Autodesk Inventor part; units mm, degrees
ref_plane "Work Plane1" through (18.5, 0, 8) normal (0, 0, 1) x (1, 0, 0)
ref_plane "YZ Plane" through (0, 0, 0) normal (1, 0, 0) x (0, 1, 0)
ref_plane "XZ Plane" through (0, 0, 0) normal (0, 1, 0) x (-1, 0, 0)
sketch "Sketch1" plane through (0, 0, 0) normal (0, 0, 1) x (1, 0, 0)
  line L0 (0, 0) -> (88, 0)
  line L1 (88, 0) -> (88, 23)
  line L2 (88, 23) -> (72, 23)
  line L3 (72, 23) -> (72, 10)
  line L4 (72, 10) -> (37, 10)
  line L5 (37, 10) -> (37, 8)
  line L6 (37, 8) -> (0, 8)
  line L7 (0, 8) -> (0, 0)
  line L8 (88, 17) -> (74, 17)
  line L9 (74, 17) -> (74, 0)
  dimension "d0" = 88
  dimension "d1" = 16
  dimension "d2" = 35
  dimension "d3" = 2
  dimension "d4" = 46
  dimension "d5" = 6
  dimension "d6" = 20
  dimension "d7" = 16
revolve "Revolution1" add sketch "Sketch1" angle 360 about axis through (0, 0, 0) along (1, 0, 0) contours L7 L6 L5 L4 L3 L2 L1 L8 L9 L0
thread "Thread1"
ref_plane "Work Plane1" through (18.5, 0, 8) normal (0, 0, 1) x (1, 0, 0)
sketch "Sketch2" plane through (18.5, 0, 8) normal (0, 0, 1) x (1, 0, 0)
  line L0 (-36.1, 0) -> (87.1, 0) construction
  line L1 (17.5, 0) -> (-0.5, 0) construction
  line L2 (15, -2.5) -> (2, -2.5)
  line L3 (2, 2.5) -> (15, 2.5)
  arc A0 (15, -2.5) -> (15, 2.5) centre (15, 0) ccw
  arc A1 (2, 2.5) -> (2, -2.5) centre (2, 0) ccw
  line L4 (18.5, -10) -> (18.5, 10)
  point P0 (-18.5, 0)
  point P1 (8.5, 0)
  point P2 (17.5, 0)
  point P3 (-0.5, 0)
  dimension "d11" = 5
  dimension "d12" = 18
  dimension "d13" = 1
extrude "Extrusion1" cut sketch "Sketch2" against normal blind 3
chamfer "Chamfer1" distance 2 angle 45 1 edges at (0, -8, 0)
properties material "Steel, Alloy"
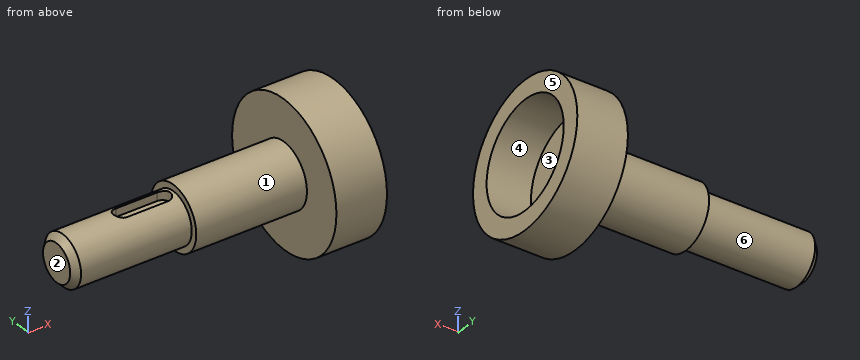
Build history of the part. All positions in model axes, mm. Face numbers are marked on the shaded views. A direction names the side the tool comes from. Coordinates: 2 decimals unless noted, no trailing zeros. Order: outer loops, then holes, each group sorted by start corner. A loop starts at its lowest first (then second) coordinate and runs counter-clockwise, first axis right, second up. Notation, with made-up numbers: M 77,-38 L 103,-38 A24 cw 103,-5 Z; hole C 6,-34 d11. An arc over 180 degrees is marked long. One line per question, with ' | ' between items. Start each with the question number.
Q1. Saw through at C-C (x = 80). List the corners of the cut face in (y, z), then the cut area to 3 significant figures.
Q2. Saw through at A-A (z = 0). List the corners of the cut face in (x, y), then the cut area to 3 significant figures.
Q3. Saw through at D-D (x = 64). List the corners of the cut face in (y, z).
Q4. Saw through at B-B (y = 0). List the corners of the cut face in (x, z).
Q5. Two-plate mould, pull along Z, no slides. Class the marked faces 4, 5 and 6: +Z half, -Z half, draft (parallel to the pull), parting line (faces both ways), or undercut.
Q6. 3-axis set-ups, long thin cutter, end or side, ignore diameter. For the marked faces 1, 2 and 3: which of +Z, -Z, +X, -X, +Y, -Y reach the whole face in a straight line?
Q7. Probe L1, parallel to Z at x = 81, y = 0; L2, parallel to X at y = -11, z = 5; L3, parallel to X at y = -7.5, z = 4.5. List the from-to ranges inside material, lowest first. Write a range as from..to.
Q8. Flat gauge pins, fed straight in: pin 1 Ø8 at (y, z) = (7.5, -5.5) entering from +X; pin 2 Ø12 at (x, y) = (60, -3) entering from +Z; pin 3 Ø5 at (x, y) = (13.5, -7) entering from +Z; pin 4 Ø4 at (x, y) = (15.5, 11.5) entering from +Z. Where does each tip first touch, or does it go through?
Check values:
1) outline: C 0,0 d46; hole C 0,0 d34 | area: 754 mm2
2) outline: M 0,-6 L 2,-8 L 37,-8 L 37,-10 L 72,-10 L 72,-23 L 88,-23 L 88,-17 L 74,-17 L 74,17 L 88,17 L 88,23 L 72,23 L 72,10 L 37,10 L 37,8 L 2,8 L 0,6 Z | area: 1,550 mm2
3) outline: C 0,0 d20
4) outline: M 0,-6 L 2,-8 L 37,-8 L 37,-10 L 72,-10 L 72,-23 L 88,-23 L 88,-17 L 74,-17 L 74,17 L 88,17 L 88,23 L 72,23 L 72,10 L 37,10 L 37,8 L 36,8 L 36,5 L 18,5 L 18,8 L 2,8 L 0,6 Z
5) face 4: undercut | face 5: draft | face 6: parting line
6) face 1: -X | face 2: +Z, -Z, -X, +Y, -Y | face 3: +X
7) L1: z = -23..-17, 17..23 | L2: x = 72..74 | L3: x = 37..74
8) pin 1: stops at x = 74 | pin 2: stops at z = 10 | pin 3: stops at z = 6.61 | pin 4: passes through
